Can you work these out from the drawing? Everything is in mm from the part's minimum corner. A direction names the side the tool comes from. Give positions to 0.01 mm unless a question says otherwise; leave off trailing zeros. Write each loop counter-clockwise with the first axis right and the second up, starting at its lowest first coordinate (ties: lowest second). Pieces come first, ordered by that corner, then holes. Notation, with made-up numbers: (49, -3.75) -> (60, -3.75) arc R25 ccw to (60, 15.25) -> close; hole circle Ø7 at (-7.75, 14). An arc over 180 degrees is marked (long way). Answer as CSV lines item,"result". Start each with the question number.
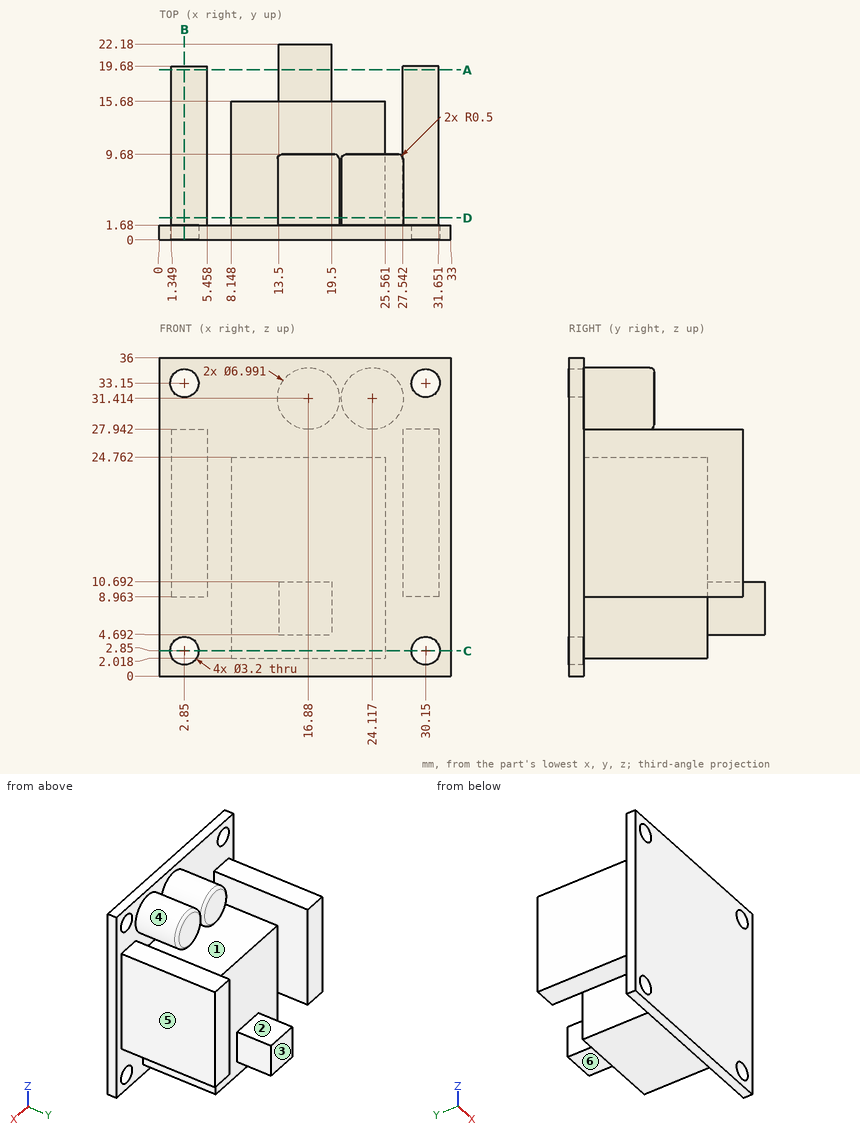
Item 1: If we section it at B-B (x = 2.85): Please give me the cut outline in (y, z), and give its area (3 significant figures).
Item 2: If we section it at A-A (y = 19.25): Please give me the cut outline in (x, z).
Item 3: If we section it at C-C (z = 2.85): Please give me the cut outline in (x, y).
Item 4: If we section it at D-D (y = 2.5): State how many separate pieces and enclosed holes the cut face has, and give its area (3 significant figures).
Item 5: We'd pull the mould along Z, two halves only. Please class the marked faces 1, 2 and 3: released by +Z, released by -Z, zero draft, split by the parting line, or undercut.
Item 6: I'm going to push flat-ended pins straight in: pin 1 (1.5 mm diameter, centred on y = 8.5, z = 14.5, fed in from -X); pin 2 (2 mm diameter, centred on x = 25.5, y = 9, fed in from +Z); pin 3 (6.5 mm diameter, centred on x = 17, z = 31, fed in from +Y); pin 4 (1.9 mm diameter, centred on x = 30.15, z = 2.85, fed in from -Y). Where does each tip first touch, or does it pass through?
Item 7: If I drill on line 1 (X direction, y = 0.9, z = 2.85); line 2 (X direction, y = 15.5, z = 20.5); line 3 (X direction, y = 11.25, z = 27), over which ranges is the centre line in solid material (lowest first)? Write a range as [from, to].
Item 8: For the marked faces 4, 5 and 6, which set-ups out of +Z, -Z, +X, -X, +Y, -Y let a thin tool reach every point of the face, with its end or its side?
Final values:
1,outline,"(0, 0) -> (1.68, 0) -> (1.68, 1.25) -> (0, 1.25) -> close; (0, 4.45) -> (1.68, 4.45) -> (1.68, 8.96) -> (19.68, 8.96) -> (19.68, 27.94) -> (1.68, 27.94) -> (1.68, 31.55) -> (0, 31.55) -> close; (0, 34.75) -> (1.68, 34.75) -> (1.68, 36) -> (0, 36) -> close"
1,area,"391 mm2"
2,outline,"(1.35, 8.96) -> (5.46, 8.96) -> (5.46, 27.94) -> (1.35, 27.94) -> close; (13.5, 4.69) -> (19.5, 4.69) -> (19.5, 10.69) -> (13.5, 10.69) -> close; (27.54, 8.96) -> (31.65, 8.96) -> (31.65, 27.94) -> (27.54, 27.94) -> close"
3,outline,"(0, 0) -> (1.25, 0) -> (1.25, 1.68) -> (0, 1.68) -> close; (4.45, 0) -> (28.55, 0) -> (28.55, 1.68) -> (25.56, 1.68) -> (25.56, 15.68) -> (8.15, 15.68) -> (8.15, 1.68) -> (4.45, 1.68) -> close; (31.75, 0) -> (33, 0) -> (33, 1.68) -> (31.75, 1.68) -> close"
4,separate pieces,"5"
4,enclosed holes,"0"
4,area,"629 mm2"
5,face 1,"undercut"
5,face 2,"released by +Z"
5,face 3,"zero draft"
6,pin 1,"x = 1.35"
6,pin 2,"z = 34.89"
6,pin 3,"y = 9.68"
6,pin 4,"through"
7,line 1,"[0, 1.25], [4.45, 28.55], [31.75, 33]"
7,line 2,"[1.35, 5.46], [8.15, 25.56], [27.54, 31.65]"
7,line 3,"[1.35, 5.46], [27.54, 31.65]"
8,face 4,"+Y"
8,face 5,"+Z, -Z, +X, +Y"
8,face 6,"-Z, +X, -X, +Y"
